```python
from build123d import *

# Parameters (mm, degrees)
F0_W     = 100
F0_H     = 100
F1_DEPTH = 1500
F2_W     = 70
F2_H     = 70
F3_DEPTH = 2001
F5_D     = 17


with BuildPart() as f1:
    # F0 (on Right) → F1 (new body)
    with BuildSketch(Plane.YZ):
        Rectangle(F0_W, F0_H)
    extrude(amount=F1_DEPTH)

    # F2 (on face) → F3 (cut)
    with BuildSketch(Plane.YZ.offset(1500)):
        Rectangle(F2_W, F2_H)
    extrude(amount=-F3_DEPTH, mode=Mode.SUBTRACT)

    # F5 (through all)
    with Locations(Plane.XZ.offset(50)):
        with Locations((250, 0), (1250, 0)):
            Hole(F5_D / 2)


solid = f1.part
```
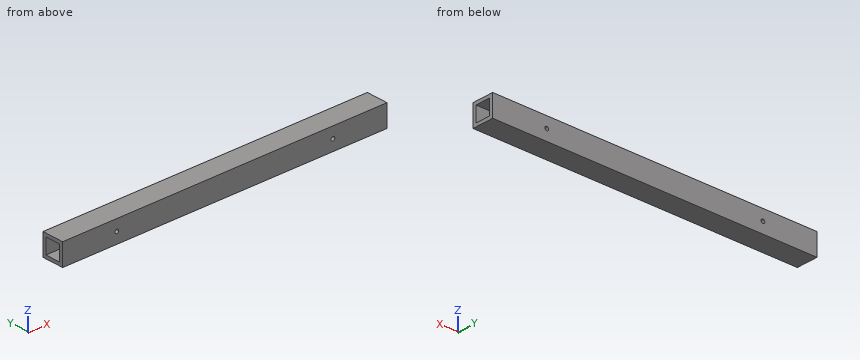
Can you work these out from the model? Positions are in its coordinate system, mm. Give positions to 0.01 mm unless a question says otherwise; leave off trailing zeros. Loops run counter-clockwise (first coordinate to the right, second up) from the corner with the lowest first, then second, coordinate; pieces in that order, holes last. Notation, with made-up numbers: M 50.5,89.5 L 94.5,89.5 A22 cw 94.5,117.5 Z; hole C 61.25,78 d4. An arc over 180 degrees is marked long. One line per question, with ' | ' between items. Start each with the question number.
Q1. If we section it at A-A (y = -17.5): Please give me the cut outline in (x, z).
Q2. If I drill on line 1 (Z direction, x = 1250, y = 40); line 2 (Y direction, x = 545, z = 17), over which ranges is the centre line in solid material (lowest first)? Write a range as from..to.
Q3. If we section it at B-B (x = 498): Please give me the cut outline in (y, z).
Computed:
1) outline: M 0,-50 L 1500,-50 L 1500,-35 L 0,-35 Z; M 0,35 L 1500,35 L 1500,50 L 0,50 Z
2) line 1: z = -50..-8.5, 8.5..50 | line 2: y = -50..-35, 35..50
3) outline: M -50,-50 L 50,-50 L 50,50 L -50,50 Z; hole M -35,-35 L 35,-35 L 35,35 L -35,35 Z
